```python
from build123d import *

# Parameters (mm, degrees)
EXTRUDE_1_DEPTH     = 15
SKETCH_2_R          = 1.5
CUT_EXTRUDE_1_DEPTH = 20


with BuildPart() as part:
    # 草图1 → 凸台-拉伸1 (new body)
    with BuildSketch(Plane.XY):
        with BuildLine():
            Line((-3, 22.405228465), (-3, 13.162446581))
            ThreePointArc((-3, 13.162446581), (-10.55343546, 8.41872912), (-13.5, 0))
            ThreePointArc((-13.5, 0), (-10.55343546, -8.41872912), (-3, -13.162446581))
            Line((-3, -13.162446581), (-3, -52.5))
            Line((-3, -52.5), (0, -52.5))
            Line((0, -52.5), (0, -12.5))
            ThreePointArc((0, -12.5), (-12.5, 0), (0, 12.5))
            Line((0, 12.5), (0, 22.405228465))
            Line((0, 22.405228465), (-3, 22.405228465))
        make_face()
    extrude(amount=EXTRUDE_1_DEPTH)

    # 草图2 → 切除-拉伸1 (cut)
    with BuildSketch(Plane.ZY.offset(3)):
        with Locations((7.5, 17.696731087)):
            Circle(SKETCH_2_R)
        with Locations((7.5, -20.291502622)):
            Circle(SKETCH_2_R)
        with Locations((7.5, -35.291502622)):
            Circle(SKETCH_2_R)
        with Locations((7.5, -45.291502622)):
            Circle(SKETCH_2_R)
    extrude(amount=-CUT_EXTRUDE_1_DEPTH, mode=Mode.SUBTRACT)


solid = part.part
```
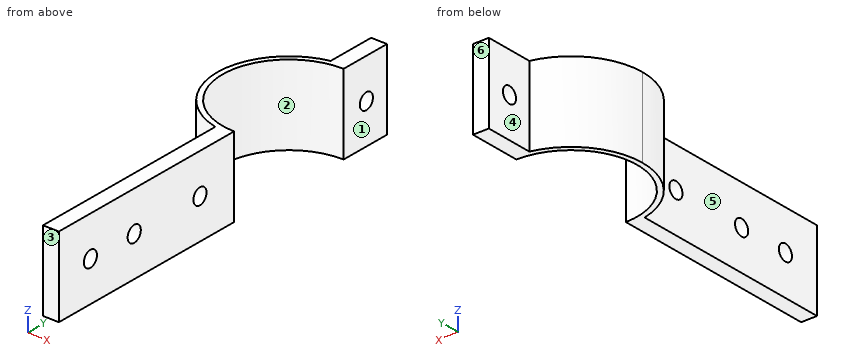
The model under review builds one solid part; all positions refer to its coordinate system, in mm. Face numbers are marked on the shaded views. A direction names the side the tool comes from. Coordinates: 2 decimals unless noted, no trailing zeros. Write each loop counter-clockwise with the first axis right and the second up, starting at its lowest first coordinate (ties: lowest second). Pieces come first, ordered by that corner, then holes.
1) We need section B-B on x = -1.5. State the section outline as (y, z) points, then the cut area to 3 significant figures.
2) The part is to be moulded in two halves that separate along Y. For the marked faces 1, 2 and 3, say which applies: pulls with the +Y half, pulls with the -Y half, needs draft (parallel to the pull), parting line crosses it, or undercut.
3) Machinability: for the marked faces 4, 5 and 6, which of the approach directions +Z, -Z, +X, -X, +Y, -Y give a long, thin tool a straight path to every point of the face, cutting with its end or side? Answer none if there is none.
4) We need section C-C on z = 4.75. State the section outline as (x, y) points.
5) We need section A-A on z = 7.5. State the section outline as (x, y) points.
6) Clearance check with flat-ended pins moving along their axes: pin 1 Ø4 at (y, z) = (-45.29, 7.5) entering from -X; pin 2 Ø2 at (x, z) = (-9, 11.5) entering from +Y; pin 3 Ø5 at (x, z) = (-8, 2.5) entering from -Y; pin 4 Ø1.8 at (y, z) = (17.7, 7.5) entering from +X. State where each tip first meets the part, or that it passes through.
7) We need section D-D on x = -4.25. State the section outline as (y, z) points, then the cut area to 3 significant figures.
8) To check wall thickness, follow probe 1 along Y at (x, z) = (-1.35, 7.5); probe 2 along Y at (x, z) = (-2.5, 7.5); probe 3 along X at (y, z) = (-18, 4). State the ranges of each line that lie inside material, in increasing order.
Answer list:
1. outline: (-52.5, 0) - (-12.41, 0) - (-12.41, 15) - (-52.5, 15) - close; (12.41, 0) - (22.41, 0) - (22.41, 15) - (12.41, 15) - close; hole circle Ø3 at (-45.29, 7.5); hole circle Ø3 at (-35.29, 7.5); hole circle Ø3 at (-20.29, 7.5); hole circle Ø3 at (17.7, 7.5)
1. area: 723 mm2
2. face 1: needs draft
2. face 2: undercut
2. face 3: pulls with the -Y half
3. face 4: +Z, -Z, -X, +Y
3. face 5: +Z, -Z, -X, -Y
3. face 6: +Z, -Z, +X, -X, +Y
4. outline: (-3, -52.5) - (0, -52.5) - (0, -12.5) arc R12.5 cw to (0, 12.5) - (0, 22.41) - (-3, 22.41) - (-3, 13.16) arc R13.5 ccw to (-3, -13.16) - close
5. outline: (-3, -52.5) - (0, -52.5) - (0, -46.79) - (-3, -46.79) - close; (-3, -43.79) - (0, -43.79) - (0, -36.79) - (-3, -36.79) - close; (-3, -33.79) - (0, -33.79) - (0, -21.79) - (-3, -21.79) - close; (-3, -18.79) - (0, -18.79) - (0, -12.5) arc R12.5 cw to (0, 12.5) - (0, 16.2) - (-3, 16.2) - (-3, 13.16) arc R13.5 ccw to (-3, -13.16) - close; (-3, 19.2) - (0, 19.2) - (0, 22.41) - (-3, 22.41) - close
6. pin 1: stops at x = -3
6. pin 2: stops at y = 10.87
6. pin 3: stops at y = -12.33
6. pin 4: passes through
7. outline: (-12.81, 0) - (-11.76, 0) - (-11.76, 15) - (-12.81, 15) - close; (11.76, 0) - (12.81, 0) - (12.81, 15) - (11.76, 15) - close
7. area: 31.7 mm2
8. probe 1: y = -52.5 to -46.79, -43.79 to -36.79, -33.79 to -21.79, -18.79 to -12.43, 12.43 to 16.2, 19.2 to 22.41
8. probe 2: y = -52.5 to -46.79, -43.79 to -36.79, -33.79 to -21.79, -18.79 to -12.25, 12.25 to 16.2, 19.2 to 22.41
8. probe 3: x = -3 to 0
